```python
from build123d import *

# Parameters (mm, degrees)
BOSS_EXTRUDE1_DEPTH = 150


with BuildPart() as part:
    # Sketch1 → Boss-Extrude1 (new body)
    with BuildSketch(Plane(origin=(0, 0, 0), x_dir=(0, 0, -1), z_dir=(1, 0, 0))):
        with BuildLine():
            Line((-17.036770748, 11.163475068), (-15.548231796, 8.558815438))
            Line((-15.548231796, 8.558815438), (-25.966870317, 2.60465963))
            Line((-25.966870317, 2.60465963), (-24.478331365, 0))
            Line((-24.478331365, 0), (-4.061294033, 11.668148498))
            ThreePointArc((-4.061294033, 11.668148498), (-2.634767864, 12.21461492), (-1.109822283, 12.304855919))
            Line((-1.109822283, 12.304855919), (22.301972464, 10.091638219))
            Line((22.301972464, 10.091638219), (22.584316562, 13.078322302))
            Line((22.584316562, 13.078322302), (10.637586676, 14.207766865))
            Line((10.637586676, 14.207766865), (10.919947816, 17.194449336))
            Line((10.919947816, 17.194449336), (-2.436908153, 18.457130406))
            ThreePointArc((-2.436908153, 18.457130406), (-3.961853734, 18.366889408), (-5.388379903, 17.820422985))
            Line((-5.388379903, 17.820422985), (-17.036770748, 11.163475068))
        make_face()
    extrude(amount=BOSS_EXTRUDE1_DEPTH)


solid = part.part
```
Read the model definition and answer for the solid it produces. Units are mm, in the model's axes. A direction names the side the tool comes from. Give positions to 0.01 mm unless a question says otherwise; leave off trailing zeros. Order: outer loops, then holes, each group sorted by start corner. A loop starts at its lowest first (then second) coordinate and runs counter-clockwise, first axis right, second up. Notation, with made-up numbers: (1.25, 88) -> (7.25, 88) arc R37 ccw to (7.25, 124) -> close; hole circle Ø3 at (61.5, 52.25). An arc over 180 degrees is marked (long way). Write item = value, one per line.
1. For faces 4 (the face through (73.95, 15.68, -10.777)), 5 (the face through (73.95, 9.879, 16.303)), 6 (the face through (73.95, 14.54, 11.13)), determine the directions among +Z, -Z, +X, -X, +Y, -Y from which every point of the face is accessible in a straight line to the end or side of a thin tool.
Numbers:
face_4 = -Z, +X, -X
face_5 = +Z, +X, -X
face_6 = +Z, +X, -X, +Y
2. A cutting plane is placed at A-A, the plane x = 133. Write down the section's boundary in (y, z).
Numbers:
outline = (0, 24.48) -> (11.67, 4.06) arc R5 cw to (12.3, 1.11) -> (10.09, -22.3) -> (13.08, -22.58) -> (14.21, -10.64) -> (17.19, -10.92) -> (18.46, 2.44) arc R5 ccw to (17.82, 5.39) -> (11.16, 17.04) -> (8.56, 15.55) -> (2.6, 25.97) -> close
3. Given pin 1 (1.5 mm diameter, centred on x = 104.5, y = 12.5, fed in from +Z); pin 2 (4 mm diameter, centred on x = 93.5, y = 8, fed in from -Z); pin 3 (8 mm diameter, centred on x = 32, z = 19, fed in from +Y); pin 4 (3 mm diameter, centred on y = 7.5, z = -15.5, fed in from -X), each flat-ended and moving along its own axis, determine where each tip first touches the part or whether it passes through.
Numbers:
pin_1 = 16.01
pin_2 = 6.98
pin_3 = 12.33
pin_4 = through
4. Straight lines are drawn through the part: line 1 along Z through (x, y) = (70.5, 14.25); line 2 along Y through (x, z) = (93, 1.5); line 3 along Y through (x, z) = (79, 14). For each, find the intervals that lie inside material, in ascending order.
Numbers:
line_1 = -10.64 to 11.64
line_2 = 12.33 to 18.37
line_3 = 5.99 to 12.9
5. The mould has two halves that part along Z. Classify faces 1 (the face through (0, 12, 4)), 2 (the face through (73.95, 18.37, 3.94)), 3 (the face through (73.95, 11.214, -10.432)): +Z half, -Z half, draft (parallel to the pull), parting line (faces both ways), or undercut.
Numbers:
face_1 = draft
face_2 = parting line
face_3 = undercut
6. A cutting plane is placed at C-C, the plane y = 5. Write down the section's boundary in (x, z).
Numbers:
outline = (0, 15.73) -> (150, 15.73) -> (150, 21.78) -> (0, 21.78) -> close
7. A cutting plane is placed at B-B, the plane z = -17. Write down the section's boundary in (x, y), and give its area (3 significant figures).
Numbers:
outline = (0, 10.59) -> (150, 10.59) -> (150, 13.61) -> (0, 13.61) -> close
area = 452 mm²
